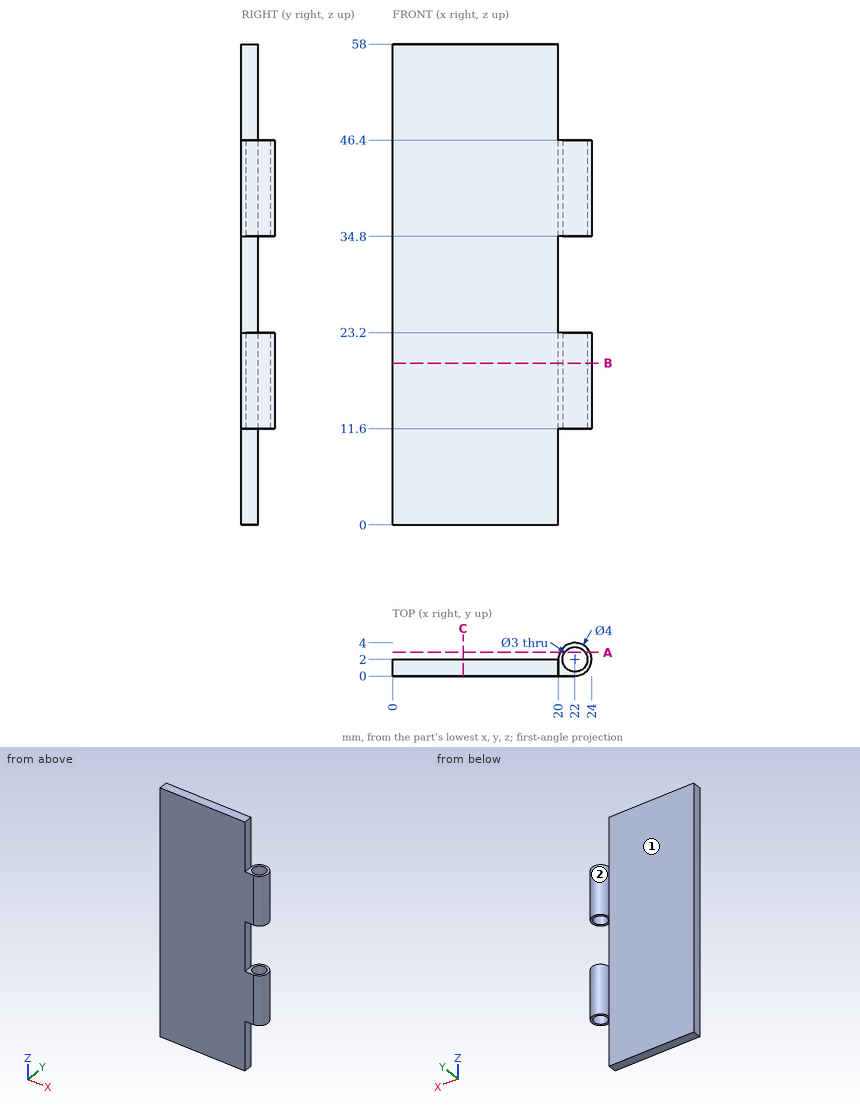
Can you work these out from the drawing? Everything is in mm from the part's minimum corner. A direction names the side the tool comes from. Coordinates: 2 decimals unless noted, no trailing zeros. Loops run counter-clockwise (first coordinate to the right, second up) from the corner with the lowest first, then second, coordinate; pieces in that order, holes last.
1. For P1, Ø6, axis at x = 5, z = 32, coming from the +Y side; P2, Ø2, axis at x = 22.5, y = 2.5, coming from the +Z side; P3, Ø2, axis at x = 21.5, y = 1, coming from the -Z side; P4, Ø1.2, axis at x = 22, y = 2.5, coming from the -Z side, each with a flat end and sliding along its axis, tell me the tip position at first contact or that it passes through.
2. For the marked faces 1 and 2, which set-ups out of +Z, -Z, +X, -X, +Y, -Y let a thin tool reach every point of the face, with its end or its side?
3. I need wall thicknesses on L1, parallel to Y at x = 22, z = 43; L2, parallel to Y at x = 1.75, z = 33; L3, parallel to X at y = 0.4, z = 46.5. Which ranges of each line are inside material? Lowest first, please.
4. Imagine slicing it at A-A, the plane y = 2.85. Please give me the cut outline in (x, z).
5. Imagine slicing it at B-B, the plane z = 19.5. Please give me the cut outline in (x, y), and give its area (3 significant figures).
6. Imagine slicing it at C-C, the plane x = 8.5. Please give me the cut outline in (y, z), and give its area (3 significant figures).
Taken from the geometry:
1. P1: stops at y = 2
1. P2: stops at z = 46.4
1. P3: stops at z = 11.6
1. P4: passes through
2. face 1: +Z, -Z, -X, +Y
2. face 2: +Z, -Z
3. L1: y = 0 to 0.5, 3.5 to 4
3. L2: y = 0 to 2
3. L3: x = 0 to 20
4. outline: (20.19, 11.6) - (20.76, 11.6) - (20.76, 23.2) - (20.19, 23.2) - close; (20.19, 34.8) - (20.76, 34.8) - (20.76, 46.4) - (20.19, 46.4) - close; (23.24, 11.6) - (23.81, 11.6) - (23.81, 23.2) - (23.24, 23.2) - close; (23.24, 34.8) - (23.81, 34.8) - (23.81, 46.4) - (23.24, 46.4) - close
5. outline: (0, 0) - (22, 0) arc R2 ccw (long way) to (20, 2) - (0, 2) - close; hole circle Ø3 at (22, 2)
5. area: 46.4 mm2
6. outline: (0, 0) - (2, 0) - (2, 58) - (0, 58) - close
6. area: 116 mm2
